Geometry: final body of the model. Coordinates: model frame, mm. Give positions to 0.01 mm unless a question says otherwise; leave off trailing zeros. Write each loop counter-clockwise with the first axis right and the second up, starting at its lowest first coordinate (ties: lowest second). Pieces come first, ordered by that corner, then holes.
```python
from build123d import *

# Parameters (mm, degrees)
SKETCH1_W           = 49
SKETCH1_H           = 15
BOSS_EXTRUDE1_DEPTH = 3
SKETCH2_R           = 3.4
CUT_EXTRUDE1_DEPTH  = 26.797286679
FILLET1_R           = 1


with BuildPart() as part:
    # Sketch1 → Boss-Extrude1 (new body)
    with BuildSketch(Plane(origin=(0, 0, 0), x_dir=(1, 0, 0), z_dir=(0, 1, 0))):
        Rectangle(SKETCH1_W, SKETCH1_H)
    extrude(amount=BOSS_EXTRUDE1_DEPTH)

    # Sketch2 → Cut-Extrude1 (cut, through all)
    with BuildSketch(Plane(origin=(0, 3, 0), x_dir=(1, 0, 0), z_dir=(0, 1, 0))):
        with Locations(Location((0, 0, 0), (0, 0, 270))):
            Circle(SKETCH2_R)
    extrude(amount=-CUT_EXTRUDE1_DEPTH, mode=Mode.SUBTRACT)

    # Fillet1
    fillet1_edges = [part.edges().sort_by_distance(p)[0] for p in [
        (-24.5, 1.5, -7.5),
        (24.5, 1.5, -7.5),
        (24.5, 1.5, 7.5),
        (-24.5, 1.5, 7.5),
    ]]
    fillet(fillet1_edges, radius=FILLET1_R)


solid = part.part
```
Item 1: Pull-direction query (Z, two-part tool) for faces 1 (the face through (24.199, 1.521, 7.215)), 2 (the face through (-3.32, 1.52, -0.74)), 3 (the face through (0, 0, -5)); classes: +Z half, -Z half, draft (parallel to the pull), parting line (faces both ways), or undercut.
Found:
face 1: +Z half
face 2: undercut
face 3: draft
Item 2: Section C-C, the plane y = 1.2. Return the cut outline in (x, z), plus the area to 3 significant figures.
Found:
outline: (-24.5, -6.5) arc R1 ccw to (-23.5, -7.5) - (23.5, -7.5) arc R1 ccw to (24.5, -6.5) - (24.5, 6.5) arc R1 ccw to (23.5, 7.5) - (-23.5, 7.5) arc R1 ccw to (-24.5, 6.5) - close; hole circle Ø6.8 at (0, 0)
area: 698 mm2
Item 3: Section A-A, the plane x = 0. Return the cut outline in (y, z), plus the area to 3 significant figures.
Found:
outline: (0, -7.5) - (3, -7.5) - (3, -3.4) - (0, -3.4) - close; (0, 3.4) - (3, 3.4) - (3, 7.5) - (0, 7.5) - close
area: 24.6 mm2
Item 4: Section B-B, the plane z = 0. Return the cut outline in (x, y).
Found:
outline: (-24.5, 0) - (-3.4, 0) - (-3.4, 3) - (-24.5, 3) - close; (3.4, 0) - (24.5, 0) - (24.5, 3) - (3.4, 3) - close
Item 5: Line query: L1, parallel to X at y = 1.3, z = 0; L2, parallel to X at y = 0.55, z = -1.25. Output: solid intervals per line, ascending.
Found:
L1: x = -24.5 to -3.4, 3.4 to 24.5
L2: x = -24.5 to -3.16, 3.16 to 24.5
